```python
from build123d import *

# Parameters (mm, degrees)
DOME1_FACE_RADIUS = 12.5
DOME1_HEIGHT      = 5


with BuildPart() as part:
    # Sketch1 → Revolve2 (revolve)
    with BuildSketch(Plane.XY, mode=Mode.PRIVATE) as revolve2_sk:
        Polygon((0, 0), (-12.5, 0), (-12.5, 30), (-13.5, 30), (-13.5, 100), (-12.5, 100), (-12.5, 160), (0, 160), align=None)
    revolve(revolve2_sk.sketch.rotate(Axis((0, 160, 0), (0, -1, 0)), 270), axis=Axis((0, 160, 0), (0, -1, 0)))

    # Dome1: a dome of height H over a round flat face of radius A is a cap of a sphere of radius (A * A + H * H) / (2 * H)
    dome1_r = (DOME1_FACE_RADIUS * DOME1_FACE_RADIUS + DOME1_HEIGHT * DOME1_HEIGHT) / (2 * DOME1_HEIGHT)
    dome1_base = Plane((0, 160, 0), z_dir=(0, 1, 0))
    with Locations(dome1_base.offset(DOME1_HEIGHT - dome1_r)):
        dome1_ball = Sphere(dome1_r, mode=Mode.PRIVATE)
    add(split(dome1_ball, bisect_by=dome1_base, keep=Keep.TOP, mode=Mode.PRIVATE))


solid = part.part
```
Here's how the part is built. I have some questions about the finished solid (model axes, mm). A direction names the side the tool comes from. Give positions to 0.01 mm unless a question says otherwise; leave off trailing zeros. Write each loop counter-clockwise with the first axis right and the second up, starting at its lowest first coordinate (ties: lowest second). Pieces come first, ordered by that corner, then holes. Notation, with made-up numbers: M -2,37 L 53,37 A27 cw 53,72 Z; hole C 8,74.5 d5. An arc over 180 degrees is marked long. Put each result on its own line as item: value. Start each with the question number.
Item 1: I need wall thicknesses on L1, parallel to Y at x = -0.5, z = 0.75; L2, parallel to Z at x = 1.5, y = 123; L3, parallel to Z at x = 10.5, y = 57.5. Which ranges of each line are inside material? Lowest first, please. Write a range as from..to.
Item 2: On a 3-axis mill with a long thin cutter (end or side, diameter ignored), from which of +Z, -Z, +X, -X, +Y, -Y can I reach the whole of each face in a straight line? I mean faces 1 (the cylindrical face through (-3.755, 15.21, 11.923)), 2 (the cylindrical face through (-3.755, 130.42, 11.923)), 3 (the cylindrical face through (13.18, 65.49, -2.93)). Say none if no direction works.
Item 3: If we section it at A-A, the plane z = 0: Write out the boundary of the cut face in (x, y) (3 decimals).
Item 4: Will these pins go through, and if not, where does the flat tip stop? pin 1 (1.5 mm diameter, centred on x = -10, y = 75.5, fed in from -Z); pin 2 (10 mm diameter, centred on x = -6.5, y = 96.5, fed in from -Z); pin 3 (1.5 mm diameter, centred on y = 36, z = -6, fed in from +X).
Item 5: If we section it at B-B, the plane x = 4.75: Write out the boundary of the cut face in (y, z) (3 decimals), then the cut area to 3 significant figures.
Item 6: If we section it at D-D, the plane y = 51.5: Write out the boundary of the cut face in (x, z), then the cut area to 3 significant figures.
Item 7: If we section it at C-C, the plane y = 122: Write out the boundary of the cut face in (x, z), then the cut area to 3 significant figures.
Values:
1. L1: 0..164.98
1. L2: -12.41..12.41
1. L3: -8.49..8.49
2. face 1: -Y
2. face 2: +Y
2. face 3: +Y, -Y
3. outline: M -13.5,30 L -12.5,30 L -12.5,0 L 12.5,0 L 12.5,30 L 13.5,30 L 13.5,100 L 12.5,100 L 12.5,160 A18.125 ccw -12.5,160 L -12.5,100 L -13.5,100 Z
4. pin 1: z = -9.83
4. pin 2: z = -13.42
4. pin 3: x = 12.44
5. outline: M 0,-11.562 L 30,-11.562 L 30,-12.637 L 100,-12.637 L 100,-11.562 L 160,-11.562 A17.492 ccw 160,11.562 L 100,11.562 L 100,12.637 L 30,12.637 L 30,11.562 L 0,11.562 Z
5. area: 3,920 mm²
6. outline: C 0,0 d27
6. area: 573 mm²
7. outline: C 0,0 d25
7. area: 491 mm²
